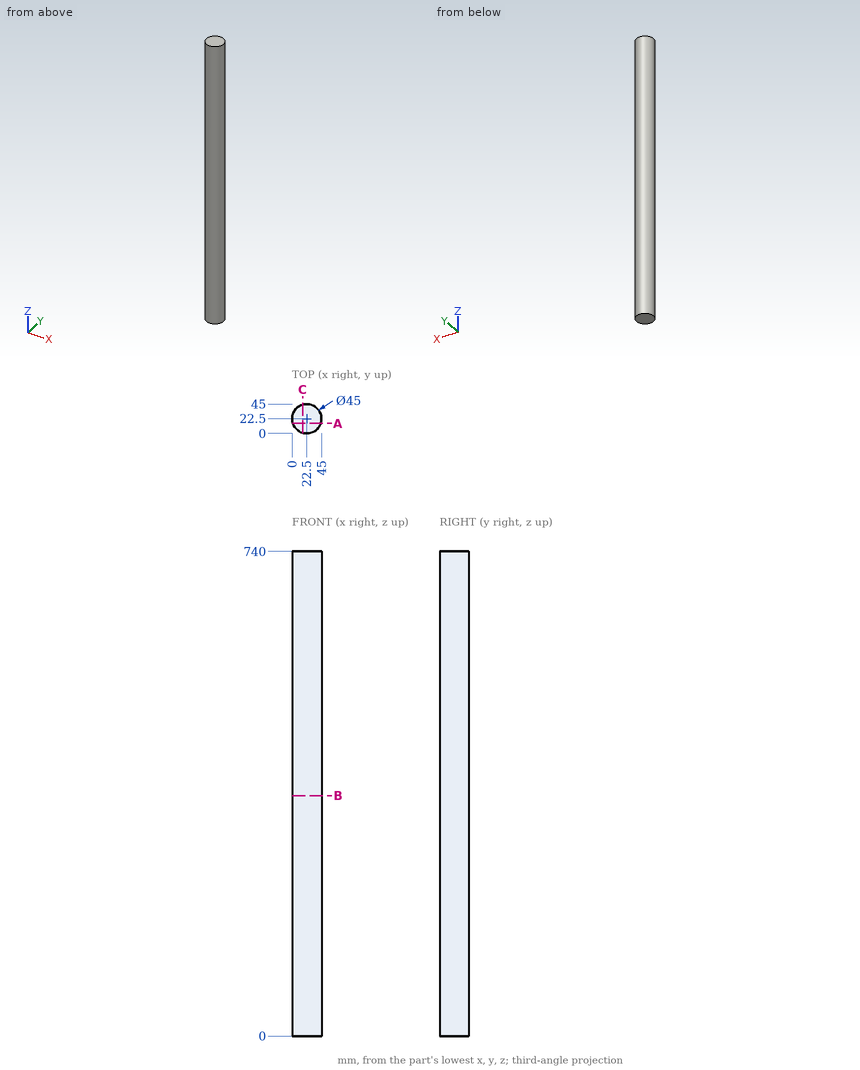
Part print with two shaded views. Sizes in mm from the minimum x, y, z corner. Round coordinates to 2 decimals unless told otherwise and drop trailing zeros. Loops run counter-clockwise (first coordinate to the right, second up) from the corner with the lowest first, then second, coordinate; pieces in that order, holes last.
Item 1: Saw through at A-A (y = 15.5). List the corners of the cut face in (x, z), then the cut area to 3 significant figures.
Item 2: Saw through at B-B (z = 367). List the corners of the cut face in (x, y), then the cut area to 3 significant figures.
Item 3: Saw through at C-C (x = 16). List the corners of the cut face in (y, z).
Item 4: Pin check, flat tips, straight feed: P1, Ø10, axis at x = 32.5, z = 238, coming from the +Y side; P2, Ø1.5, axis at y = 12, z = 170, coming from the +X side; P3, Ø1.5, axis at x = 7.5, z = 167, coming from the -Y side. Stop position of each tip, or through.
Item 5: Drill centre lines: line 1 along X through (y, z) = (24.5, 547); line 2 along X through (y, z) = (36, 190); line 3 along Y through (x, z) = (5.5, 504.5). Where is each one in solid material? Low to high.
Worked answers:
1. outline: (1.12, 0) - (43.88, 0) - (43.88, 740) - (1.12, 740) - close
1. area: 31,600 mm2
2. outline: circle Ø45 at (22.5, 22.5)
2. area: 1,590 mm2
3. outline: (0.96, 0) - (44.04, 0) - (44.04, 740) - (0.96, 740) - close
4. P1: stops at y = 44.44
4. P2: stops at x = 42.78
4. P3: stops at y = 5.09
5. line 1: x = 0.09 to 44.91
5. line 2: x = 4.5 to 40.5
5. line 3: y = 7.76 to 37.24
